```python
from build123d import *

# Parameters (mm, degrees)
BOSS_EXTRUDE1_DEPTH = 65
FILLET1_R           = 8
CUT_EXTRUDE1_DEPTH  = 65
CUT_EXTRUDE2_REACH  = 177.118
CUT_EXTRUDE3_DEPTH  = 50


with BuildPart() as part:
    # Sketch1 → Boss-Extrude1 (new body)
    with BuildSketch(Plane(origin=(0, 0, 0), x_dir=(1, 0, 0), z_dir=(0, 1, 0))):
        Polygon((-75.055534995, 0.197193855), (-37.527767497, -64.802806145), (37.527767497, -64.802806145), (75.055534995, 0.197193855), (37.527767497, 65.197193855), (-37.527767497, 65.197193855), align=None)
    extrude(amount=BOSS_EXTRUDE1_DEPTH)

    # Fillet1
    fillet1_edges = [part.edges().sort_by_distance(p)[0] for p in [
        (-37.527767497, 32.5, -65.197193855),
        (37.527767497, 32.5, -65.197193855),
        (75.055534995, 32.5, -0.197193855),
        (37.527767497, 32.5, 64.802806145),
        (-37.527767497, 32.5, 64.802806145),
        (-75.055534995, 32.5, -0.197193855),
    ]]
    fillet(fillet1_edges, radius=FILLET1_R)

    # Sketch2 → Cut-Extrude1 (cut)
    with BuildSketch(Plane(origin=(0, 0, 0), x_dir=(1, 0, 0), z_dir=(0, 1, 0))):
        Polygon((-39.707247658, 51.225029628), (-24.769507731, 60), (24.508553139, 60), (39.576770362, 51.451022934), (64.215800796, 8.774970372), (64.346278093, -8.548977066), (39.707247658, -51.225029628), (24.769507731, -60), (-24.508553139, -60), (-39.576770362, -51.451022934), (-64.215800796, -8.774970372), (-64.346278093, 8.548977066), align=None)
    extrude(amount=CUT_EXTRUDE1_DEPTH, mode=Mode.SUBTRACT)

    # Cut-Extrude2: up to this face of the body (flat: up to its plane)
    cut_extrude2_end = Plane(part.part.faces().sort_by_distance((56.291651246, 32.5, -32.697193855))[0])
    # Sketch4 → Cut-Extrude2 (cut, up to the picked face)
    with BuildSketch(Plane(origin=(-56.206263802, 0, 32.450701536), x_dir=(0.5000000000000002, 0, 0.8660254037844386), z_dir=(-0.8660254037844386, 0, 0.5000000000000002)), mode=Mode.PRIVATE) as cut_extrude2_sk1:
        with BuildLine():
            Line((-4.64838762, 31.756705854), (-25.916422712, 12.61547427))
            ThreePointArc((-25.916422712, 12.61547427), (-26.992226029, 12.445268353), (-27.585387444, 13.358768416))
            Line((-27.585387444, 13.358768416), (-27.585387444, 51.641231584))
            ThreePointArc((-27.585387444, 51.641231584), (-26.992226029, 52.554731647), (-25.916422712, 52.38452573))
            Line((-25.916422712, 52.38452573), (-4.64838762, 33.243294146))
            ThreePointArc((-4.64838762, 33.243294146), (-4.317352351, 32.5), (-4.64838762, 31.756705854))
        make_face()
    cut_extrude2_tool1 = split(extrude(cut_extrude2_sk1.sketch, amount=-CUT_EXTRUDE2_REACH, mode=Mode.PRIVATE), bisect_by=cut_extrude2_end, keep=Keep.BOTH, mode=Mode.PRIVATE)
    # Sketch4 → Cut-Extrude2 (cut, up to the picked face)
    with BuildSketch(Plane(origin=(-56.206263802, 0, 32.450701536), x_dir=(0.5000000000000002, 0, 0.8660254037844386), z_dir=(-0.8660254037844386, 0, 0.5000000000000002)), mode=Mode.PRIVATE) as cut_extrude2_sk2:
        with BuildLine():
            Line((-0.754352176, 36.46547427), (-21.63349838, 55.256705854))
            ThreePointArc((-21.63349838, 55.256705854), (-21.89815406, 56.358263767), (-20.964533648, 57))
            Line((-20.964533648, 57), (20.79375876, 57))
            ThreePointArc((20.79375876, 57), (21.727379172, 56.358263767), (21.462723491, 55.256705854))
            Line((21.462723491, 55.256705854), (0.583577288, 36.46547427))
            ThreePointArc((0.583577288, 36.46547427), (-0.085387444, 36.208768416), (-0.754352176, 36.46547427))
        make_face()
    cut_extrude2_tool2 = split(extrude(cut_extrude2_sk2.sketch, amount=-CUT_EXTRUDE2_REACH, mode=Mode.PRIVATE), bisect_by=cut_extrude2_end, keep=Keep.BOTH, mode=Mode.PRIVATE)
    # Sketch4 → Cut-Extrude2 (cut, up to the picked face)
    with BuildSketch(Plane(origin=(-56.206263802, 0, 32.450701536), x_dir=(0.5000000000000002, 0, 0.8660254037844386), z_dir=(-0.8660254037844386, 0, 0.5000000000000002)), mode=Mode.PRIVATE) as cut_extrude2_sk3:
        with BuildLine():
            Line((21.462723491, 9.743294146), (0.583577288, 28.53452573))
            ThreePointArc((0.583577288, 28.53452573), (-0.085387444, 28.791231584), (-0.754352176, 28.53452573))
            Line((-0.754352176, 28.53452573), (-21.63349838, 9.743294146))
            ThreePointArc((-21.63349838, 9.743294146), (-21.89815406, 8.641736233), (-20.964533648, 8))
            Line((-20.964533648, 8), (20.79375876, 8))
            ThreePointArc((20.79375876, 8), (21.727379172, 8.641736233), (21.462723491, 9.743294146))
        make_face()
    cut_extrude2_tool3 = split(extrude(cut_extrude2_sk3.sketch, amount=-CUT_EXTRUDE2_REACH, mode=Mode.PRIVATE), bisect_by=cut_extrude2_end, keep=Keep.BOTH, mode=Mode.PRIVATE)
    # Sketch4 → Cut-Extrude2 (cut, up to the picked face)
    with BuildSketch(Plane(origin=(-56.206263802, 0, 32.450701536), x_dir=(0.5000000000000002, 0, 0.8660254037844386), z_dir=(-0.8660254037844386, 0, 0.5000000000000002)), mode=Mode.PRIVATE) as cut_extrude2_sk4:
        with BuildLine():
            Line((25.640806472, 52.519982346), (4.473644042, 33.267260514))
            ThreePointArc((4.473644042, 33.267260514), (4.146519039, 32.52223718), (4.481455433, 31.780692745))
            Line((4.481455433, 31.780692745), (25.849775962, 12.751479913))
            ThreePointArc((25.849775962, 12.751479913), (26.926458787, 12.586929236), (27.514811958, 13.503533499))
            Line((27.514811958, 13.503533499), (27.313653858, 51.785468163))
            ThreePointArc((27.313653858, 51.785468163), (26.715700577, 52.695838803), (25.640806472, 52.519982346))
        make_face()
    cut_extrude2_tool4 = split(extrude(cut_extrude2_sk4.sketch, amount=-CUT_EXTRUDE2_REACH, mode=Mode.PRIVATE), bisect_by=cut_extrude2_end, keep=Keep.BOTH, mode=Mode.PRIVATE)
    add(cut_extrude2_tool1.solids().sort_by(Axis((-66.026454, 32.5, 15.441634), (0.8660254037844386, 0, -0.5000000000000002)))[0], mode=Mode.SUBTRACT)
    add(cut_extrude2_tool2.solids().sort_by(Axis((-56.248958, 49.92174, 32.376754), (0.8660254037844386, 0, -0.5000000000000002)))[0], mode=Mode.SUBTRACT)
    add(cut_extrude2_tool3.solids().sort_by(Axis((-56.248958, 15.07826, 32.376754), (0.8660254037844386, 0, -0.5000000000000002)))[0], mode=Mode.SUBTRACT)
    add(cut_extrude2_tool4.solids().sort_by(Axis((-46.471596, 32.602753, 49.31164), (0.8660254037844386, 0, -0.5000000000000002)))[0], mode=Mode.SUBTRACT)

    # Sketch6 → Cut-Extrude3 (cut)
    with BuildSketch(Plane(origin=(-56.206263802, 0, -32.845089247), x_dir=(0.5, 0, -0.8660254037844386), z_dir=(0.8660254037844387, 0, 0.5000000000000001))):
        with BuildLine():
            Line((-4.64838762, 31.756705854), (-25.916422712, 12.61547427))
            ThreePointArc((-25.916422712, 12.61547427), (-26.992226029, 12.445268353), (-27.585387444, 13.358768416))
            Line((-27.585387444, 13.358768416), (-27.585387444, 51.641231584))
            ThreePointArc((-27.585387444, 51.641231584), (-26.992226029, 52.554731647), (-25.916422712, 52.38452573))
            Line((-25.916422712, 52.38452573), (-4.64838762, 33.243294146))
            ThreePointArc((-4.64838762, 33.243294146), (-4.317352351, 32.5), (-4.64838762, 31.756705854))
        make_face()
        with BuildLine():
            Line((-0.754352176, 36.46547427), (-21.63349838, 55.256705854))
            ThreePointArc((-21.63349838, 55.256705854), (-21.89815406, 56.358263767), (-20.964533648, 57))
            Line((-20.964533648, 57), (20.79375876, 57))
            ThreePointArc((20.79375876, 57), (21.727379172, 56.358263767), (21.462723491, 55.256705854))
            Line((21.462723491, 55.256705854), (0.583577288, 36.46547427))
            ThreePointArc((0.583577288, 36.46547427), (-0.085387444, 36.208768416), (-0.754352176, 36.46547427))
        make_face()
        with BuildLine():
            Line((21.462723491, 9.743294146), (0.583577288, 28.53452573))
            ThreePointArc((0.583577288, 28.53452573), (-0.085387444, 28.791231584), (-0.754352176, 28.53452573))
            Line((-0.754352176, 28.53452573), (-21.63349838, 9.743294146))
            ThreePointArc((-21.63349838, 9.743294146), (-21.89815406, 8.641736233), (-20.964533648, 8))
            Line((-20.964533648, 8), (20.79375876, 8))
            ThreePointArc((20.79375876, 8), (21.727379172, 8.641736233), (21.462723491, 9.743294146))
        make_face()
        with BuildLine():
            Line((25.640806472, 52.519982346), (4.473644042, 33.267260514))
            ThreePointArc((4.473644042, 33.267260514), (4.146519039, 32.52223718), (4.481455433, 31.780692745))
            Line((4.481455433, 31.780692745), (25.849775962, 12.751479913))
            ThreePointArc((25.849775962, 12.751479913), (26.926458787, 12.586929236), (27.514811958, 13.503533499))
            Line((27.514811958, 13.503533499), (27.313653858, 51.785468163))
            ThreePointArc((27.313653858, 51.785468163), (26.715700577, 52.695838803), (25.640806472, 52.519982346))
        make_face()
    extrude(amount=CUT_EXTRUDE3_DEPTH, mode=Mode.SUBTRACT)


solid = part.part
```
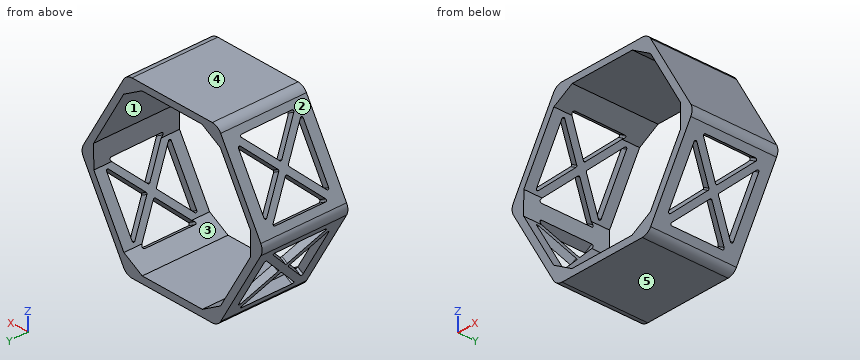
Work out the finished part from the listing and answer in its coordinate system (mm). Face numbers are marked on the shaded views. A direction names the side the tool comes from. Round coordinates to 2 decimals unless told otherwise and drop trailing zeros. Write each loop counter-clockwise with the first axis right and the second up, starting at its lowest first coordinate (ties: lowest second). Pieces come first, ordered by that corner, then holes.
1) Consider probe 1 along Z at (x, y) = (10.5, 15); probe 2 along X at (y, z) = (46, -17); probe 3 along Z at (x, y) = (59, 27). Determine where each line is inside the solid, lowest interval first.
2) Determine the mould class of the marked faces 3, 4 and 5 for opening direction Z: pulls with the +Z half, pulls with the -Z half, needs draft (parallel to the pull), parting line crosses it, or undercut.
3) A cutting plane is placed at A-A on x = 7. Determine the outline of the cut face in (y, z).
4) A cutting plane is placed at C-C on y = 25. Give the number of separate pieces and of enclosed holes in the cut face, and give its area (3 significant figures).
5) A cutting plane is placed at B-B on z = 19.5. Determine the outline of the cut face in (x, y), and give its area (3 significant figures).
6) Which of the six approach directions +Z, -Z, +X, -X, +Y, -Y give full straight-line access (tool end or side, diameter ignored) to the marked faces 1 and 2?
7) Flat-ended cylindrical pins translate along their axes: P1, Ø8, axis at x = -39, y = 35, coming from the +Z side; P2, Ø7.5, axis at x = -58.5, z = 22.5, coming from the -Y side; P3, Ø10, axis at y = 14.5, z = 34.5, coming from the -X side; P4, Ø3, axis at y = 45.5, z = -18.5, coming from the -X side. Find the tip coordinate at first contact, or state that the pin passes through.
Entries:
1. probe 1: z = -65.2 to -60, 60 to 64.8
1. probe 2: x = -65.35 to -59.47, 59.47 to 65.35
1. probe 3: z = -28.01 to -22.69, 17.81 to 27.61
2. face 3: undercut
2. face 4: pulls with the +Z half
2. face 5: pulls with the -Z half
3. outline: (0, -65.2) - (65, -65.2) - (65, -60) - (0, -60) - close; (0, 60) - (65, 60) - (65, 64.8) - (0, 64.8) - close
4. separate pieces: 9
4. enclosed holes: 0
4. area: 1,790 mm2
5. outline: (-63.68, 0) - (-58.02, 0) - (-58.02, 8) - (-63.68, 8) - close; (-63.68, 15.75) - (-58.02, 18.3) - (-58.02, 25.03) - (-63.68, 22.48) - close; (-63.68, 42.52) - (-58.02, 39.97) - (-58.02, 46.7) - (-63.68, 49.25) - close; (-63.68, 57) - (-58.02, 57) - (-58.02, 65) - (-63.68, 65) - close; (58.02, 0) - (63.68, 0) - (63.68, 65) - (58.02, 65) - close
5. area: 535 mm2
6. face 1: +Y, -Y
6. face 2: +Z, -X, +Y, -Y
7. P1: stops at z = 64.52
7. P2: stops at y = 0
7. P3: stops at x = 46.48
7. P4: stops at x = -65.35
